The figure shows three views and two pictorial views of one solid part (mm, origin at its lowest corner). Answer the questions. Coordinates: 2 decimals unless noted, no trailing zeros. Write each loop counter-clockwise with the first axis right and the second up, starting at its lowest first coordinate (ties: lowest second). Pieces come first, ordered by that corner, then holes.
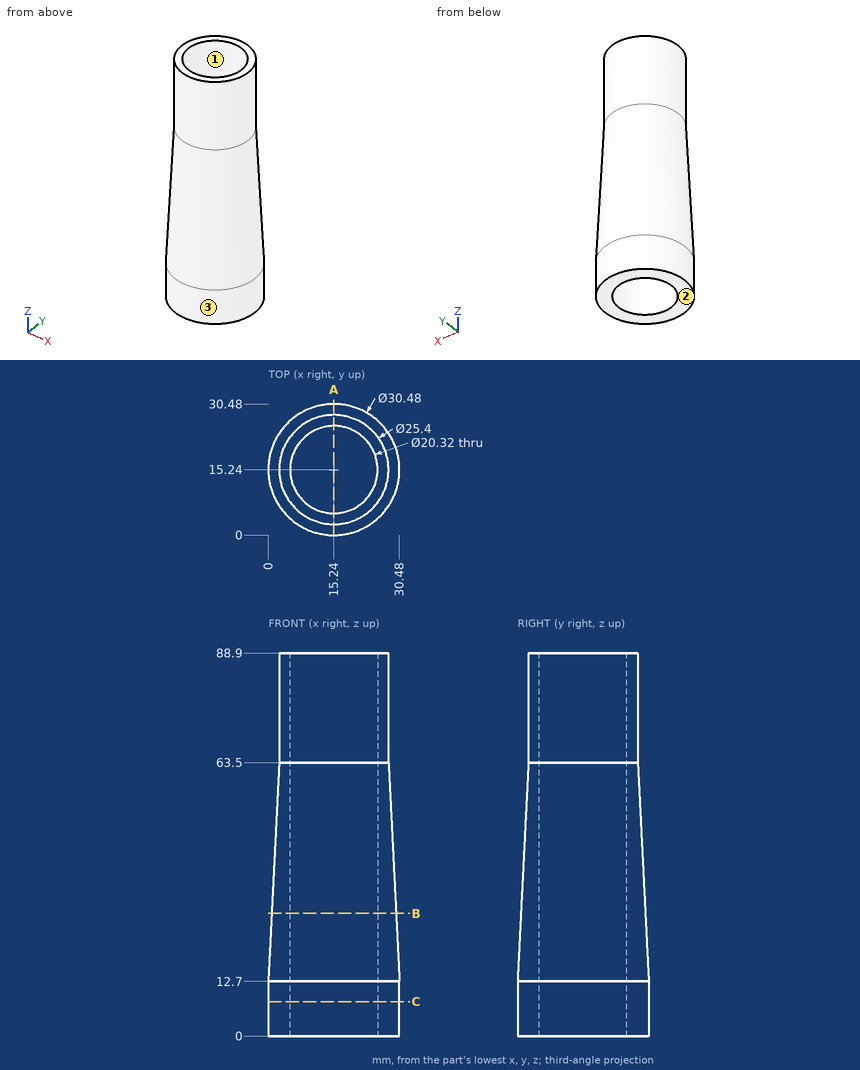
Q1. The part is cut by section A-A, the plane x = 15.24. Write down the section's boundary in (y, z), then the cut area to 3 significant figures.
Answers below:
outline: (0, 0) - (5.08, 0) - (5.08, 88.9) - (2.54, 88.9) - (2.54, 63.5) - (0, 12.7) - close; (25.4, 0) - (30.48, 0) - (30.48, 12.7) - (27.94, 63.5) - (27.94, 88.9) - (25.4, 88.9) - close
area: 645 mm2
Q2. Find the intervals of material crossed by probe 1 along X at (y, z) = (15, 29); probe 2 along Y at (x, z) = (15, 51); probe 3 along X at (y, z) = (6, 69), in increasing order.
Answers below:
probe 1: x = 0.82 to 5.08, 25.4 to 29.66
probe 2: y = 1.92 to 5.08, 25.4 to 28.56
probe 3: x = 6.53 to 11.02, 19.46 to 23.95
Q3. Given pin 1 (6 mm diameter, centred on y = 21, z = 13, fed in from -X); pin 2 (1 mm diameter, centred on y = 3.5, z = 45, fed in from +X); pin 3 (10 mm diameter, centred on x = 12.5, z = 20, fed in from -Y), each flat-ended and moving along its own axis, determine where each tip first touches the part or whether it passes through.
Answers below:
pin 1: stops at x = 0.25
pin 2: stops at x = 22.94
pin 3: stops at y = 0.15
Q4. The part is cut by section C-C, the plane z = 8. Write down the section's boundary in (x, y), then the cut area to 3 significant figures.
Answers below:
outline: circle Ø30.48 at (15.24, 15.24); hole circle Ø20.32 at (15.24, 15.24)
area: 405 mm2
Q5. Determine the mould class of the marked faces 1, 2 and 3 for opening direction X: released by +X, released by -X, zero draft, split by the parting line, or undercut.
Answers below:
face 1: undercut
face 2: zero draft
face 3: split by the parting line
Q6. The part is cut by section B-B, the plane z = 28.5. Write down the section's boundary in (x, y).
Answers below:
outline: circle Ø28.9 at (15.24, 15.24); hole circle Ø20.32 at (15.24, 15.24)
